For this review, take the finished solid that the model builds, in its own axes (mm). A direction names the side the tool comes from. Coordinates: 2 decimals unless noted, no trailing zeros. Loops run counter-clockwise (first coordinate to the right, second up) from the corner with the lowest first, then second, coordinate; pieces in that order, holes last. Notation, with made-up numbers: M 78,9.5 L 82,9.5 A11 cw 82,25.5 Z; hole C 84,-7 d3. An arc over 180 degrees is marked long. Use one line per item in the form item = value.
```python
from build123d import *

# Parameters (mm, degrees)
BOSS_EXTRUDE1_DEPTH = 2
BOSS_EXTRUDE2_START = 2
SKETCH2_R           = 3.65
BOSS_EXTRUDE2_DEPTH = 2
SKETCH3_R           = 3.5
CUT_EXTRUDE1_DEPTH  = 2


with BuildPart() as part:
    # Sketch1 → Boss-Extrude1 (new body)
    with BuildSketch(Plane(origin=(0, 0, 0), x_dir=(1, 0, 0), z_dir=(0, 1, 0))):
        with BuildLine():
            Line((-3.57318314, -7.255109239), (-2, 8))
            ThreePointArc((-2, 8), (0, 10), (2, 8))
            Line((2, 8), (3.57318314, -7.255109239))
            ThreePointArc((3.57318314, -7.255109239), (0, -11.65), (-3.57318314, -7.255109239))
        make_face()
    extrude(amount=-BOSS_EXTRUDE1_DEPTH)

    # Sketch2 → Boss-Extrude2 (add)
    with BuildSketch(Plane(origin=(0, 0, 0), x_dir=(1, 0, 0), z_dir=(0, 1, 0)).offset(BOSS_EXTRUDE2_START)):
        with Locations(Location((0, -8, 0), (0, 0, 270))):
            Circle(SKETCH2_R)
    extrude(amount=-BOSS_EXTRUDE2_DEPTH)

    # Sketch3 → Cut-Extrude1 (cut)
    with BuildSketch(Plane(origin=(0, 2, 0), x_dir=(1, 0, 0), z_dir=(0, 1, 0))):
        with Locations(Location((0, -8, 0), (0, 0, 270))):
            Circle(SKETCH3_R)
    extrude(amount=-CUT_EXTRUDE1_DEPTH, mode=Mode.SUBTRACT)


solid = part.part
```
1. Wall thickness on line 1 along X through (y, z) = (0.65, 8); line 2 along Y through (x, z) = (2, 4.75); line 3 along X through (y, z) = (1.8, 6.25): over which ranges is each line inside the solid? List them lowest first. Write a range as from..to.
Computed values:
line_1 = -3.65..-3.5, 3.5..3.65
line_2 = -2..0
line_3 = -3.2..-3.03, 3.03..3.2
2. Consider section C-C on y = 1.45. Write out the cut boundary in (x, z).
Computed values:
outline = C 0,8 d7.3; hole C 0,8 d7
3. Consider section B-B on x = -1.5. Write out the cut boundary in (y, z).
Computed values:
outline = M -2,-9.32 L 0,-9.32 L 0,4.67 L 2,4.67 L 2,4.84 L 0,4.84 L 0,11.16 L 2,11.16 L 2,11.33 L -2,11.33 Z
4. Consider section D-D on x = -3. Write out the cut boundary in (y, z), plus the area to 3 significant figures.
Computed values:
outline = M -2,1.7 L 0,1.7 L 0,5.92 L 2,5.92 L 2,6.2 L 0,6.2 L 0,9.8 L 2,9.8 L 2,10.08 L -2,10.08 Z
area = 17.9 mm2
5. For pin 1 Ø1 at (x, y) = (-1.5, -0.5) entering from -Z; pin 2 Ø2 at (x, y) = (2.5, 1.5) entering from -Z, all flat-tipped, find the tip position at first contact; note any pin that passes through.
Computed values:
pin_1 = -9.73
pin_2 = 4.67
6. Tool access review of faces 4 (the face through (0, -1, -10)), 5 (the face through (0, 0, 8)): name each direction out of +Z, -Z, +X, -X, +Y, -Y from which nothing blocks a thin tool from reaching the whole face with its end or side.
Computed values:
face_4 = -Z, +Y, -Y
face_5 = +Y
7. Consider section A-A on z = 8. Write out the cut boundary in (x, y).
Computed values:
outline = M -3.65,-2 L 3.65,-2 L 3.65,2 L 3.5,2 L 3.5,0 L -3.5,0 L -3.5,2 L -3.65,2 Z
8. Draft analysis for pull direction Z (two halves, no side actions). For faces 1 (the face through (0, -2, 1)), 2 (the face through (-2.1, 1, 5.2)), 3 (the face through (-2.798, -0.986, -0.266)), state which applies: +Z half, -Z half, draft (parallel to the pull), parting line (faces both ways), or undercut.
Computed values:
face_1 = draft
face_2 = undercut
face_3 = -Z half
